Verification items for the finished model (mm, model axes). Face numbers are marked on the shaded views. A direction names the side the tool comes from. Coordinates: 2 decimals unless noted, no trailing zeros. Loops run counter-clockwise (first coordinate to the right, second up) from the corner with the lowest first, then second, coordinate; pieces in that order, holes last. Notation, with made-up numbers: (64, 58) -> (80, 58) arc R26 ccw to (80, 80) -> close; hole circle Ø7 at (21, 80). An arc over 180 degrees is marked (long way). Answer as a JSON object with one key per item and string values. Group by question number.
Q1. Set-up check for the marked faces 5 and 6: record each of +Z, -Z, +X, -X, +Y, -Y from which the full face is reachable in a straight line by a thin tool's end or side.
Q2. Cross-section at D-D on x = 36.5. Record the boundary of the cut face in (y, z), and give its area (3 significant figures).
Q3. Cross-section at C-C on z = 4.1. Record the boundary of the cut face in (x, y) (1 decimal), and give its area (3 significant figures).
Q4. Release check for a two-part mould opening along Y. For the marked faces 1, 2, 3 and 4 record: released by +Y, released by -Y, zero draft, split by the parting line, or undercut.
Q5. Cross-section at A-A on x = 0. Record the boundary of the cut face in (y, z), and give its area (3 significant figures).
Q6. Scan lines: L1, parallel to Y at x = 0, z = 3.4; L2, parallel to X at y = 0, z = 1.1; L3, parallel to X at y = -13, z = 1.9. Record each from-to range of solid material in increasing order.
Q7. Cross-section at B-B on y = 5. Record the boundary of the cut face in (x, z), and give its area (3 significant figures).
Q8. Gauge pin test, flat end, axial feed: pin 1 Ø1 at (x, z) = (-33, 3.5) entering from +Y. Record the tip position at first contact, or that the pin passes through.
```python
from build123d import *

# Parameters (mm, degrees)
F1_DEPTH = 5
F2_R     = 30
F4_DEPTH = 5.001
F5_R     = 30
F6_R     = 30
F7_R     = 5
F8_R     = 5
F9_R     = 5
F10_R    = 5


with BuildPart() as f1:
    # F0 (on Top) → F1 (new body)
    with BuildSketch(Plane.XY):
        with BuildLine():
            Line((-42.497829, -10.052536), (-37.314063, -19.814464))
            ThreePointArc((-37.314063, -19.814464), (37.956578, -18.553988), (-7.285654, 41.615761))
            Line((-7.285654, 41.615761), (-14.006471, 44.062227))
            Line((-14.006471, 44.062227), (-21.715557, 42.017373))
            Line((-21.715557, 42.017373), (-28.90164, 34.610507))
            Line((-28.90164, 34.610507), (-30.980071, 27.070666))
            Line((-30.980071, 27.070666), (-29.551746, 24.139418))
            Line((-29.551746, 24.139418), (-40.117525, 13.249019))
            Line((-40.117525, 13.249019), (-42.248696, 0))
            Line((-42.248696, 0), (-42.497829, -10.052536))
        make_face()
        with BuildLine():
            ThreePointArc((-5.28408, 32.384846), (26.613249, -19.194653), (-32.397266, -5.207392))
            Line((-32.397266, -5.207392), (-32.397266, 10.650216))
            Line((-32.397266, 10.650216), (-28.90164, 23.331157))
            Line((-28.90164, 23.331157), (-25.874414, 22.175578))
            Line((-25.874414, 22.175578), (-14.777807, 22.175578))
            Line((-14.777807, 22.175578), (-7.285654, 27.070666))
            Line((-7.285654, 27.070666), (-5.28408, 32.384846))
        make_face(mode=Mode.SUBTRACT)
    extrude(amount=F1_DEPTH)

    # F2
    f2_edges = [f1.edges().sort_by_distance(p)[0] for p in [
        (-42.497829, -10.052536, 2.5),
    ]]
    fillet(f2_edges, radius=F2_R)

    # F3 (on face) → F4 (cut, through all)
    with BuildSketch(Plane.XY.offset(5)):
        Polygon((-33.602018, 2.287856), (-32.397266, -5.207392), (-32.397266, 10.650216), align=None)
    extrude(amount=-F4_DEPTH, mode=Mode.SUBTRACT)

    # F5
    f5_edges = [f1.edges().sort_by_distance(p)[0] for p in [
        (-40.117525, 13.249019, 2.5),
    ]]
    fillet(f5_edges, radius=F5_R)

    # F6
    f6_edges = [f1.edges().sort_by_distance(p)[0] for p in [
        (-33.602018, 2.287856, 2.5),
    ]]
    fillet(f6_edges, radius=F6_R)

    # F7
    f7_edges = [f1.edges().sort_by_distance(p)[0] for p in [
        (-30.980071, 27.070666, 2.5),
    ]]
    fillet(f7_edges, radius=F7_R)

    # F8
    f8_edges = [f1.edges().sort_by_distance(p)[0] for p in [
        (-25.874414, 22.175578, 2.5),
    ]]
    fillet(f8_edges, radius=F8_R)

    # F9
    f9_edges = [f1.edges().sort_by_distance(p)[0] for p in [
        (-28.90164, 34.610507, 2.5),
        (-21.715557, 42.017373, 2.5),
        (-14.006471, 44.062227, 2.5),
    ]]
    fillet(f9_edges, radius=F9_R)

    # F10
    f10_edges = [f1.edges().sort_by_distance(p)[0] for p in [
        (-14.777807, 22.175578, 2.5),
        (-7.285654, 27.070666, 2.5),
    ]]
    fillet(f10_edges, radius=F10_R)


solid = f1.part
```
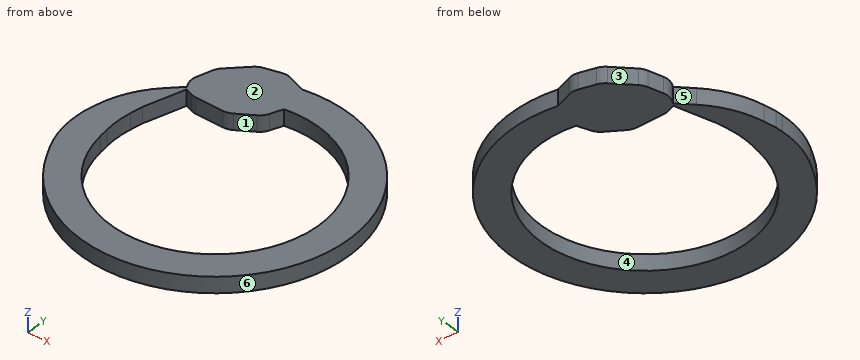
Computed values:
{
 "1": {"face 5": "+Z, -Z, -X", "face 6": "+Z, -Z"},
 "2": {"outline": "(-21.28, 0) -> (21.28, 0) -> (21.28, 5) -> (-21.28, 5) -> close", "area": "213 mm²"},
 "3": {"outline": "(-42.3, -2.2) arc R30 ccw to (-38.8, -17) -> (-37.3, -19.8) arc R42.2 ccw (long way) to (-7.3, 41.6) -> (-12.5, 43.5) arc R5 ccw to (-15.5, 43.7) -> (-20.4, 42.4) arc R5 ccw to (-22.7, 41) -> (-28, 35.5) arc R5 ccw to (-29.2, 33.4) -> (-30.5, 28.9) arc R5 ccw to (-30.2, 25.4) -> (-29.6, 24.1) -> (-33.5, 20) arc R30 ccw to (-41.6, 3.9) -> (-42.2, 0) -> close; hole (-33, 6.8) arc R30 ccw to (-32.9, -2.2) -> (-32.4, -5.2) arc R32.8 ccw (long way) to (-5.3, 32.4) -> (-6.7, 28.6) arc R5 cw to (-8.7, 26.2) -> (-13.5, 23) arc R5 cw to (-16.3, 22.2) -> (-25, 22.2) arc R5 cw to (-26.7, 22.5) -> (-28.9, 23.3) -> (-32.4, 10.7) -> close", "area": "2,310 mm²"},
 "4": {"face 1": "undercut", "face 2": "zero draft", "face 3": "released by +Y", "face 4": "undercut"},
 "5": {"outline": "(-42.25, 0) -> (-32.81, 0) -> (-32.81, 5) -> (-42.25, 5) -> close; (32.81, 0) -> (42.25, 0) -> (42.25, 5) -> (32.81, 5) -> close", "area": "94.4 mm²"},
 "6": {"L1": "y = -42.25 to -32.81, 32.81 to 42.25", "L2": "x = -42.25 to -33.15, 32.81 to 42.25", "L3": "x = -40.57 to -30.13, 30.13 to 40.2"},
 "7": {"outline": "(-41.42, 0) -> (-33.16, 0) -> (-33.16, 5) -> (-41.42, 5) -> close; (32.43, 0) -> (41.95, 0) -> (41.95, 5) -> (32.43, 5) -> close", "area": "89.0 mm²"},
 "8": {"pin 1": "stops at y = 21.1"}
}
